Autodesk Inventor part; units mm, degrees
ref_plane "YZ Plane" through (0, 0, 0) normal (1, 0, 0) x (0, 1, 0)
ref_plane "XZ Plane" through (0, 0, 0) normal (0, 1, 0) x (-1, 0, 0)
ref_plane "XY Plane" through (0, 0, 0) normal (0, 0, 1) x (1, 0, 0)
sketch "Sketch1" plane through (0, 0, 0) normal (0, 0, 1) x (1, 0, 0)
  line L0 (-25, -25) -> (25, -25)
  line L1 (25, -25) -> (25, 25)
  line L2 (25, 25) -> (-25, 25)
  line L3 (-25, 25) -> (-25, -25)
  point P0 (0, 0)
  dimension "d0" = 50
  dimension "d1" = 50
  dimension "d2" = 25
  dimension "d3" = 25
extrude "Extrusion1" add sketch "Sketch1" along normal blind 150
sketch "Sketch2" plane through (0, 0, 0) normal (0, 0, -1) x (-1, 0, 0)
  circle A0 centre (0, 0) radius 5
  dimension "d6" = 10
extrude "Extrusion2" add sketch "Sketch2" along normal blind 10
sketch "Sketch3" plane through (0, 0, 150) normal (0, 0, 1) x (1, 0, 0)
  line L0 (-200, -12.5) -> (0, -12.5)
  line L1 (0, -12.5) -> (0, 12.5)
  line L2 (0, 12.5) -> (-200, 12.5)
  line L3 (-200, 12.5) -> (-200, -12.5)
  line L4 (-200, -350) -> (-175, -350)
  line L5 (-175, -350) -> (-175, 350)
  line L6 (-175, 350) -> (-200, 350)
  line L7 (-200, 350) -> (-200, -350)
  line L8 (200, -12.5) -> (0, -12.5)
  line L9 (0, 12.5) -> (200, 12.5)
  line L10 (200, 12.5) -> (200, -12.5)
  line L11 (200, -350) -> (175, -350)
  line L12 (175, -350) -> (175, 350)
  line L13 (175, 350) -> (200, 350)
  line L14 (200, 350) -> (200, -350)
  point P0 (0, 0)
  point P1 (0, 0)
  point P2 (-187.5, -350)
  point P3 (187.5, -350)
  point P4 (-175, -12.5)
  point P5 (175, -12.5)
  point P6 (175, 12.5)
  point P7 (-175, 12.5)
  dimension "d9" = 25
  dimension "d10" = 200
  dimension "d11" = 25
  dimension "d12" = 700
  dimension "d13" = 350
extrude "Extrusion3" add sketch "Sketch3" along normal blind 50
sketch "Sketch4" plane through (0, 0, 200) normal (0, 0, 1) x (1, 0, 0)
  line L0 (-200, -350) -> (-175, -350)
  circle A0 centre (-187.5, -350) radius 60
  line L1 (-187.5, -350) -> (-187.5, 371.532) construction
  line L2 (-187.5, -350) -> (187.5, -350) construction
  line L3 (175, -350) -> (200, -350)
  circle A1 centre (-187.5, 350) radius 60
  circle A2 centre (187.5, -350) radius 60
  circle A3 centre (187.5, 350) radius 60
  point P0 (0, 0)
  dimension "d16" = 120
  dimension "d19" = 700
  dimension "d22" = 375
extrude "Extrusion4" add sketch "Sketch4" along normal blind 25
equation "\"d0\" = d1"
properties part number "LINK 6"
Here's how the part is built. I have some questions about the finished solid (model axes, mm). A direction names the side the tool comes from. Round coordinates to 2 decimals unless told otherwise and drop trailing zeros. Loops run counter-clockwise (first coordinate to the right, second up) from the corner with the lowest first, then second, coordinate; pieces in that order, holes last.
1. For P1, Ø15, axis at y = -244, z = 186, coming from the -X side; P2, Ø20, axis at x = 187.5, z = 166, coming from the -Y side; P3, Ø8, axis at y = 15, z = 27, coming from the -X side, each with a flat end and sliding along its axis, tell me the tip position at first contact or that it passes through.
Answer list:
P1: stops at x = -200
P2: stops at y = -350
P3: stops at x = -25
2. Which directions (+Z, -Z, +X, -X, +Y, -Y) give clear straight access to the entire face, cutting with the end or side of a thin tool? Please do faces 1 (the face through (25, 0, 74)), 2 (the face through (0, -25, 74)), 3 (the face through (-187, 350, 175)), 4 (the face through (-1, 1, 200)), 5 (the face through (-175, -184, 175)).
Answer list:
face 1: -Z, +X, +Y, -Y
face 2: +Z, -Z, +X, -X, -Y
face 3: -Z, +X, -X, +Y
face 4: +Z, +X, -X
face 5: -Z, -Y
3. If I drill on line 1 along X through (y, z) = (-340.5, 158.5); line 2 along Y through (x, z) = (72.5, 170.5); line 3 along Y through (x, z) = (197.5, 175.5), over which ranges is the centre line in solid material (lowest first)?
Answer list:
line 1: x = -200 to -175, 175 to 200
line 2: y = -12.5 to 12.5
line 3: y = -350 to 350
4. We'd pull the mould along X, two halves only. Please class faces 6 (the face through (175, -184, 175)), 7 (the face through (-188, 351, 200)), 8 (the face through (-188, 351, 225)), 9 (the face through (200, 5, 175)): +X half, -X half, draft (parallel to the pull), parting line (faces both ways), or undercut.
Answer list:
face 6: undercut
face 7: undercut
face 8: draft
face 9: +X half
5. If we section it at D-D on y = -311.5: Write out the boundary of the cut face in (x, z), plus the area to 3 significant figures.
Answer list:
outline: (-233.52, 200) - (-200, 200) - (-200, 150) - (-175, 150) - (-175, 200) - (-141.48, 200) - (-141.48, 225) - (-233.52, 225) - close; (141.48, 200) - (175, 200) - (175, 150) - (200, 150) - (200, 200) - (233.52, 200) - (233.52, 225) - (141.48, 225) - close
area: 7,100 mm2
6. If we section it at B-B on z = 163: Write out the boundary of the cut face in (x, y), plus the area to 4 significant figures.
Answer list:
outline: (-200, -350) - (-175, -350) - (-175, -12.5) - (175, -12.5) - (175, -350) - (200, -350) - (200, 350) - (175, 350) - (175, 12.5) - (-175, 12.5) - (-175, 350) - (-200, 350) - close
area: 43,750 mm2
7. If we section it at C-C on x = 187.5: Write out the boundary of the cut face in (y, z).
Answer list:
outline: (-410, 200) - (-350, 200) - (-350, 150) - (350, 150) - (350, 200) - (410, 200) - (410, 225) - (290, 225) - (290, 200) - (-290, 200) - (-290, 225) - (-410, 225) - close
8. If we section it at A-A on y = 215: Write out the boundary of the cut face in (x, z).
Answer list:
outline: (-200, 150) - (-175, 150) - (-175, 200) - (-200, 200) - close; (175, 150) - (200, 150) - (200, 200) - (175, 200) - close
